from build123d import *

# Parameters (mm, degrees)
SKETCH_1_R      = 1.6
EXTRUDE_1_DEPTH = 5
FILLET_1_R      = 5


with BuildPart() as part:
    # 草图1 → 凸台-拉伸1 (new body)
    with BuildSketch(Plane.XY):
        Polygon((-67.081805701, 36.641915025), (-2.081805701, 36.641915025), (-2.081805701, 71.641915025), (117.918194299, 71.641915025), (117.918194299, 36.641915025), (182.918194299, 36.641915025), (182.918194299, -113.358084975), (117.918194299, -113.358084975), (117.918194299, -148.358084975), (-2.081805701, -148.358084975), (-2.081805701, -113.358084975), (-67.081805701, -113.358084975), align=None)
        with Locations((-49.081283258, 29.641915025)):
            Circle(SKETCH_1_R, mode=Mode.SUBTRACT)
        with Locations((-19.081283258, 29.673445995)):
            Circle(SKETCH_1_R, mode=Mode.SUBTRACT)
        with Locations((-49.060066678, 5.641915025)):
            Circle(SKETCH_1_R, mode=Mode.SUBTRACT)
        with Locations((-19.081283258, 5.673445995)):
            Circle(SKETCH_1_R, mode=Mode.SUBTRACT)
        with Locations(Location((164.896455276, 5.641915025, 0), (0, 0, 180))):
            Circle(SKETCH_1_R, mode=Mode.SUBTRACT)
        with Locations(Location((134.917671856, 5.673445995, 0), (0, 0, 180))):
            Circle(SKETCH_1_R, mode=Mode.SUBTRACT)
        with Locations(Location((134.917671856, 29.673445995, 0), (0, 0, 180))):
            Circle(SKETCH_1_R, mode=Mode.SUBTRACT)
        with Locations(Location((164.917671856, 29.641915025, 0), (0, 0, 180))):
            Circle(SKETCH_1_R, mode=Mode.SUBTRACT)
        with Locations((134.917671856, -82.389615946)):
            Circle(SKETCH_1_R, mode=Mode.SUBTRACT)
        with Locations((164.896455276, -82.358084975)):
            Circle(SKETCH_1_R, mode=Mode.SUBTRACT)
        with Locations((164.917671856, -106.358084975)):
            Circle(SKETCH_1_R, mode=Mode.SUBTRACT)
        with Locations((134.917671856, -106.389615946)):
            Circle(SKETCH_1_R, mode=Mode.SUBTRACT)
        with Locations(Location((-49.060066678, -82.358084975, 0), (0, 0, 180))):
            Circle(SKETCH_1_R, mode=Mode.SUBTRACT)
        with Locations(Location((-19.081283258, -82.389615946, 0), (0, 0, 180))):
            Circle(SKETCH_1_R, mode=Mode.SUBTRACT)
        with Locations(Location((-19.081283258, -106.389615946, 0), (0, 0, 180))):
            Circle(SKETCH_1_R, mode=Mode.SUBTRACT)
        with Locations(Location((-49.081283258, -106.358084975, 0), (0, 0, 180))):
            Circle(SKETCH_1_R, mode=Mode.SUBTRACT)
    extrude(amount=EXTRUDE_1_DEPTH)

    # 圆角1
    fillet_1_edges = [part.edges().sort_by_distance(p)[0] for p in [
        (-67.081805701, 36.641915025, 2.5),
        (-2.081805701, 71.641915025, 2.5),
        (117.918194299, 71.641915025, 2.5),
        (182.918194299, 36.641915025, 2.5),
        (182.918194299, -113.358084975, 2.5),
        (117.918194299, -148.358084975, 2.5),
        (-2.081805701, -148.358084975, 2.5),
        (-67.081805701, -113.358084975, 2.5),
    ]]
    fillet(fillet_1_edges, radius=FILLET_1_R)


solid = part.part
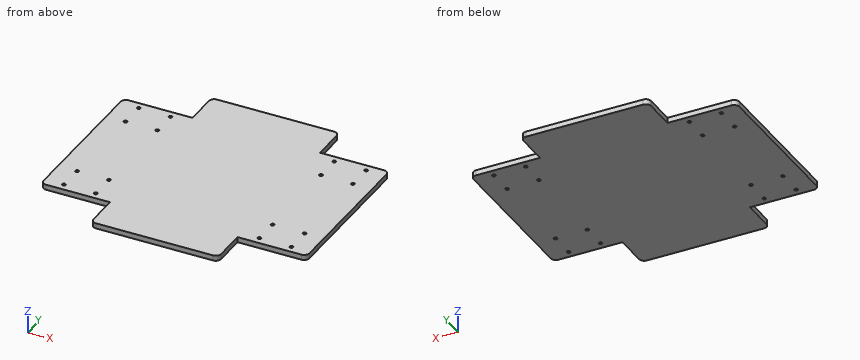
Could you check a few things on this model? Use its own coordinates, in mm. Round coordinates to 2 decimals unless told otherwise and drop trailing zeros. Loops run counter-clockwise (first coordinate to the right, second up) from the corner with the lowest first, then second, coordinate; pieces in that order, holes last. Notation, with made-up numbers: (82.25, 19) - (137.25, 19) arc R12 ccw to (137.25, 35) - close; hole circle Ø11 at (45, 31.25). An arc over 180 degrees is marked (long way). Write item = value, one per line.
1) I'm going to push flat-ended pins straight in: P1, Ø1.9, axis at x = 134.92, y = 5.67, coming from the -Z side; P2, Ø2, axis at y = -126, z = 2.5, coming from the -X side; P3, Ø2.5, axis at x = -39.5, z = 2, coming from the -Y side. Where does each tip first touch, or does it pass through?
Computed:
P1 = through
P2 = -2.08
P3 = -113.36
2) Imagine slicing it at B-B (z = 3.6). Give the number of separate pieces and of enclosed holes in the cut face, and give its area (3 significant figures).
Computed:
separate_pieces = 1
enclosed_holes = 16
area = 45,700 mm2
3) Imagine slicing it at A-A (y = -117). Please give me the cut outline in (x, z), and give its area (3 significant figures).
Computed:
outline = (-2.08, 0) - (117.92, 0) - (117.92, 5) - (-2.08, 5) - close
area = 600 mm2
4) I need wall thicknesses on line 1 along Y through (x, z) = (135, 4.5); line 2 along Y through (x, z) = (-24, 1.3); line 3 along Y through (x, z) = (-18, 2.6). Which ranges of each line are inside material? Lowest first, please. Write a range as from..to.
Computed:
line_1 = -113.36..-107.99, -104.79..-83.99, -80.79..4.08, 7.27..28.08, 31.27..36.64
line_2 = -113.36..36.64
line_3 = -113.36..-107.57, -105.21..-83.57, -81.21..4.49, 6.85..28.49, 30.85..36.64
